Autodesk Inventor part; units mm, degrees
ref_plane "YZ Plane" through (0, 0, 0) normal (1, 0, 0) x (0, 1, 0)
ref_plane "XZ Plane" through (0, 0, 0) normal (0, 1, 0) x (-1, 0, 0)
ref_plane "XY Plane" through (0, 0, 0) normal (0, 0, 1) x (1, 0, 0)
sketch "Sketch4" plane through (0, 0, 0) normal (0, 0, 1) x (1, 0, 0)
  line L0 (0, 0) -> (150, 0)
  line L1 (150, 0) -> (150, 150)
  line L2 (150, 150) -> (0, 150)
  line L3 (0, 150) -> (0, 0)
  dimension "d34" = 150
  dimension "d35" = 150
extrude "Extrusion4" add sketch "Sketch4" along normal blind 10
sketch "Sketch5" plane through (0, 0, 10) normal (0, 0, 1) x (1, 0, 0)
  line L0 (10, 10) -> (140, 10)
  line L1 (140, 10) -> (140, 140)
  line L2 (140, 140) -> (10, 140)
  line L3 (10, 140) -> (10, 10)
  point P0 (0, 0)
  dimension "d38" = 130
  dimension "d39" = 130
extrude "Extrusion5" cut sketch "Sketch5" against normal blind 2
sketch "Sketch6" plane through (0, 0, 0) normal (0, 0, -1) x (-1, 0, 0)
  circle A0 centre (-75, 75) radius 14.35
  circle A1 centre (-75, 75) radius 17.15
  line L0 (-147.5, 2.5) -> (-142.5, 2.5)
  line L1 (-142.5, 2.5) -> (-142.5, 7.5)
  line L2 (-142.5, 7.5) -> (-147.5, 7.5)
  line L3 (-147.5, 7.5) -> (-147.5, 2.5)
  line L4 (-2.5, 2.5) -> (-7.5, 2.5)
  line L5 (-7.5, 2.5) -> (-7.5, 7.5)
  line L6 (-7.5, 7.5) -> (-2.5, 7.5)
  line L7 (-2.5, 7.5) -> (-2.5, 2.5)
  line L8 (-147.5, 147.5) -> (-142.5, 147.5)
  line L9 (-142.5, 147.5) -> (-142.5, 142.5)
  line L10 (-142.5, 142.5) -> (-147.5, 142.5)
  line L11 (-147.5, 142.5) -> (-147.5, 147.5)
  line L12 (-2.5, 147.5) -> (-7.5, 147.5)
  line L13 (-7.5, 147.5) -> (-7.5, 142.5)
  line L14 (-7.5, 142.5) -> (-2.5, 142.5)
  line L15 (-2.5, 142.5) -> (-2.5, 147.5)
  point P0 (0, 0)
  dimension "d42" = 28.7
  dimension "d43" = 34.3
  dimension "d46" = 5
  dimension "d47" = 5
  dimension "d48" = 5
  dimension "d49" = 5
  dimension "d50" = 5
  dimension "d51" = 5
  dimension "d52" = 5
  dimension "d53" = 5
extrude "Extrusion7" cut sketch "Sketch6" against normal blind 5
sketch "Sketch7" plane through (0, 0, 8) normal (0, 0, 1) x (1, 0, 0)
  line L0 (47.5, 102.5) -> (102.5, 102.5)
  line L1 (102.5, 102.5) -> (102.5, 47.5)
  line L2 (102.5, 47.5) -> (47.5, 47.5)
  line L3 (47.5, 47.5) -> (47.5, 102.5)
  point P0 (0, 0)
  dimension "d58" = 55
  dimension "d59" = 55
extrude "Extrusion8" cut sketch "Sketch7" against normal blind 2
sketch "Sketch9" plane through (0, 0, 6) normal (0, 0, 1) x (1, 0, 0)
  line L0 (47.5, 47.5) -> (47.5, 102.5)
  line L1 (47.5, 47.5) -> (102.5, 47.5)
  line L2 (102.5, 47.5) -> (102.5, 102.5)
  line L3 (102.5, 102.5) -> (47.5, 102.5)
  line L4 (47.5, 102.5) -> (47.5, 47.5)
  point P0 (0, 0)
  dimension "d68" = 55
  dimension "d69" = 55
extrude "Extrusion10" add sketch "Sketch9" along normal blind 2
sketch "Sketch10" plane through (0, 0, 8) normal (0, 0, 1) x (1, 0, 0)
  line L0 (37.5, 37.5) -> (112.5, 37.5)
  line L1 (112.5, 37.5) -> (112.5, 112.5)
  line L2 (37.5, 37.5) -> (112.5, 37.5)
  line L3 (112.5, 37.5) -> (112.5, 112.5)
  line L4 (112.5, 112.5) -> (37.5, 112.5)
  line L5 (37.5, 112.5) -> (37.5, 37.5)
  point P0 (0, 0)
  dimension "d72" = 75
  dimension "d73" = 75
extrude "Extrusion11" add sketch "Sketch10" along normal blind 5
sketch "Sketch11" plane through (0, 0, 13) normal (0, 0, 1) x (1, 0, 0)
  line L0 (47.5, 47.5) -> (102.5, 47.5)
  line L1 (102.5, 47.5) -> (102.5, 102.5)
  line L2 (102.5, 102.5) -> (47.5, 102.5)
  line L3 (47.5, 102.5) -> (47.5, 47.5)
  point P0 (0, 0)
  dimension "d76" = 55
  dimension "d77" = 55
extrude "Extrusion12" cut sketch "Sketch11" against normal blind 2
sketch "Sketch12" plane through (0, 0, 11) normal (0, 0, 1) x (1, 0, 0)
  circle A0 centre (75, 75) radius 14.35
  circle A1 centre (75, 75) radius 17.15
  point P0 (0, 0)
sketch "Sketch13" plane through (0, 0, 8) normal (0, 0, 1) x (1, 0, 0)
  line L0 (140, 140) -> (140, 10)
  line L1 (10, 140) -> (140, 140)
  line L2 (140, 140) -> (140, 10)
  line L3 (140, 10) -> (10, 10)
  line L4 (10, 10) -> (10, 140)
  line L5 (37.5, 37.5) -> (37.5, 112.5)
  line L6 (112.5, 112.5) -> (112.5, 37.5)
  line L7 (37.5, 112.5) -> (112.5, 112.5)
  line L8 (112.5, 112.5) -> (112.5, 37.5)
  line L9 (112.5, 37.5) -> (37.5, 37.5)
  line L10 (37.5, 37.5) -> (37.5, 112.5)
  point P0 (0, 0)
extrude "Extrusion13" add sketch "Sketch13" along normal blind 5
sketch "Sketch15" plane through (0, 0, 10) normal (0, 0, 1) x (1, 0, 0)
  line L0 (0, 0) -> (150, 0)
  line L1 (150, 0) -> (150, 150)
  line L2 (150, 150) -> (0, 150)
  line L3 (0, 150) -> (0, 0)
  line L4 (10, 140) -> (10, 10)
  line L5 (10, 140) -> (140, 140)
  line L6 (140, 140) -> (140, 10)
  line L7 (140, 10) -> (10, 10)
  line L8 (10, 10) -> (10, 140)
  dimension "d86" = 150
  dimension "d87" = 150
  dimension "d88" = 130
  dimension "d89" = 130
extrude "Extrusion14" add sketch "Sketch15" along normal blind 5
properties part number "Elbow_Both_Marker_TestFit_V2"
Geometry: final body of the model. Coordinates: model frame, mm. A direction names the side the tool comes from. Give positions to 0.01 mm unless a question says otherwise; leave off trailing zeros. Order: outer loops, then holes, each group sorted by start corner. A loop starts at its lowest first (then second) coordinate and runs counter-clockwise, first axis right, second up. Notation, with made-up numbers: (-9, 19) - (34, 19) arc R26 cw to (34, 39) - close; hole circle Ø8 at (6.5, 51). An arc over 180 degrees is marked (long way). Use CSV: the item, a comma, the result in double quotes.
1. Section query C-C (y = 100.5). Output: boundary loops of the cut face in (x, z).
Answers below:
outline,"(0, 0) - (150, 0) - (150, 15) - (140, 15) - (140, 13) - (102.5, 13) - (102.5, 11) - (47.5, 11) - (47.5, 13) - (10, 13) - (10, 15) - (0, 15) - close"
2. Section query A-A (x = 75). Output: boundary loops of the cut face in (y, z).
Answers below:
outline,"(0, 0) - (57.85, 0) - (57.85, 5) - (60.65, 5) - (60.65, 0) - (89.35, 0) - (89.35, 5) - (92.15, 5) - (92.15, 0) - (150, 0) - (150, 15) - (140, 15) - (140, 13) - (102.5, 13) - (102.5, 11) - (47.5, 11) - (47.5, 13) - (10, 13) - (10, 15) - (0, 15) - close"
3. Section query D-D (x = 20.5). Output: boundary loops of the cut face in (y, z), plus the area to 3 significant figures.
Answers below:
outline,"(0, 0) - (150, 0) - (150, 15) - (140, 15) - (140, 13) - (10, 13) - (10, 15) - (0, 15) - close"
area,"1,990 mm2"
4. Contact query for flat-ended pins moving along their axis: pin 1 (2 mm diameter, centred on x = 126, y = 109, fed in from +Z); pin 2 (2.5 mm diameter, centred on x = 145, y = 144, fed in from -Z). Output: stop coordinate, or through.
Answers below:
pin 1,"z = 13"
pin 2,"z = 5"
5. Mould query, pull axis Y, two halves, no side actions, for faces 1 (the face through (76, 150, 7)), 2 (the face through (5, 5, 5)), 3 (the face through (141, 76, 15)), 4 (the face through (5, 142.5, 2)). Classes: +Y half, -Y half, draft (parallel to the pull), parting line (faces both ways), or undercut.
Answers below:
face 1,"+Y half"
face 2,"undercut"
face 3,"draft"
face 4,"undercut"
6. Material intervals for line 1 along Y through (x, z) = (75, 1.65); line 2 along X through (y, z) = (21, 14); line 3 along Y through (x, z) = (60, 12), sorted ascending. Write a range as from..to.
Answers below:
line 1,"0..57.85, 60.65..89.35, 92.15..150"
line 2,"0..10, 140..150"
line 3,"0..47.5, 102.5..150"
7. Access query for faces 5 (the face through (5, 7.5, 2)), 6 (the face through (0, 76, 7)). Directions: +Z, -Z, +X, -X, +Y, -Y. A direction counts if a zero-diameter tool reaches every point of the face in a straight line with its end or side. Return the directions, or none.
Answers below:
face 5,"-Z"
face 6,"+Z, -Z, -X, +Y, -Y"
